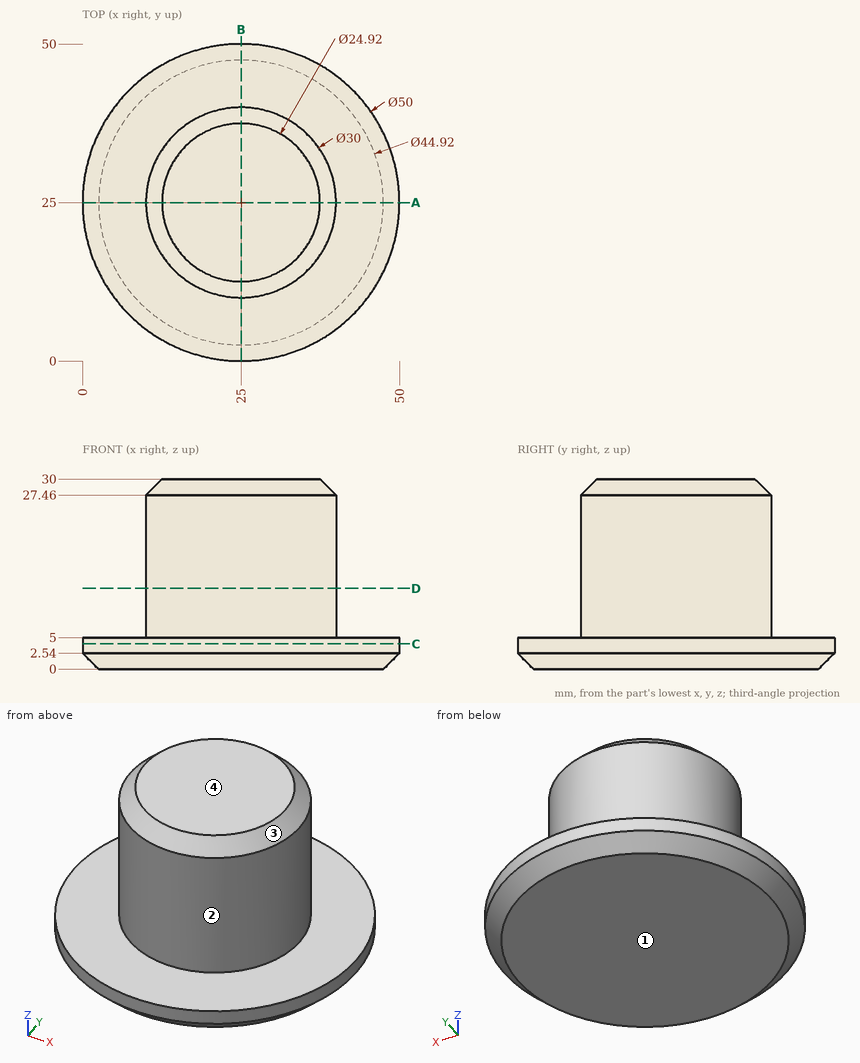
Drawing for the job (mm, zero at the part's lowest x, y, z). A direction names the side the tool comes from. Give positions to 0.01 mm unless a question says otherwise; leave off trailing zeros. Loops run counter-clockwise (first coordinate to the right, second up) from the corner with the lowest first, then second, coordinate; pieces in that order, holes last.
Item 1: Slice it at D-D (z = 12.75). Write the cut outline in (x, y).
Check values:
outline: circle Ø30 at (25, 25)
Item 2: Which spindle directions (+Z, -Z, +X, -X, +Y, -Y) get a long thin tool onto all of the face, cutting with end or side? Do the marked faces 1 and 2. Say none if no direction does.
Check values:
face 1: -Z, +X, -X, +Y, -Y
face 2: +Z
Item 3: Slice it at C-C (z = 4). Write the cut outline in (x, y).
Check values:
outline: circle Ø50 at (25, 25)
Item 4: Mould opens along Y. For the marked faces 3 and 4 say: +Y half, -Y half, draft (parallel to the pull), parting line (faces both ways), or undercut.
Check values:
face 3: parting line
face 4: draft
Item 5: Slice it at A-A (y = 25). Write the cut outline in (x, z), plus the area to 3 significant figures.
Check values:
outline: (0, 2.54) - (2.54, 0) - (47.46, 0) - (50, 2.54) - (50, 5) - (40, 5) - (40, 27.46) - (37.46, 30) - (12.54, 30) - (10, 27.46) - (10, 5) - (0, 5) - close
area: 987 mm2
Item 6: Drill centre lines: line 1 along Z through (x, y) = (30, 41); line 2 along Y through (x, z) = (17.5, 24.5); line 3 along Z through (x, y) = (39, 22). Where is each one in solid material? Low to high.
Check values:
line 1: z = 0 to 5
line 2: y = 12.01 to 37.99
line 3: z = 0 to 28.14
Item 7: Drop flat-ended pins along their axis: P1, Ø8, axis at x = 30.5, z = 3.5, coming from the +Y side; P2, Ø6, axis at x = 30.5, z = 27, coming from the -Y side; P3, Ø12, axis at y = 35, z = 7.5, coming from the -X side. Give the stop position or say it passes through.
Check values:
P1: stops at y = 49.95
P2: stops at y = 10.21
P3: stops at x = 0.42
